For this review, take the finished solid that the model builds, in its own axes (mm). A direction names the side the tool comes from. Give positions to 0.01 mm unless a question says otherwise; leave off trailing zeros. Order: outer loops, then holes, each group sorted by start corner. A loop starts at its lowest first (then second) coordinate and runs counter-clockwise, first axis right, second up. Notation, with made-up numbers: (32.25, 68.25) - (58.25, 68.25) arc R21 ccw to (58.25, 83.25) - close; hole circle Ø4 at (79.5, 26.25). An arc over 180 degrees is marked (long way). Put each result on its own line as item: value. Start each with the question number.
```python
from build123d import *

# Parameters (mm, degrees)
BOSS_EXTRUDE1_DEPTH = 5
SKETCH2_R           = 2
CUT_EXTRUDE1_DEPTH  = 7
SKETCH3_R           = 2
CUT_EXTRUDE2_DEPTH  = 7
FILLET1_R           = 3


with BuildPart() as part:
    # Sketch1 → Boss-Extrude1 (new, symmetric)
    with BuildSketch(Plane.XY):
        with BuildLine():
            Line((0, 32), (0, 0))
            Line((0, 0), (8, 0))
            ThreePointArc((8, 0), (22.296085696, 3.651940128), (37, 4.880613018))
            ThreePointArc((37, 4.880613018), (49.464275388, 0.752368163), (57, -10))
            Line((57, -10), (65, -10))
            Line((65, -10), (65, 22))
            Line((65, 22), (57, 22))
            ThreePointArc((57, 22), (42.703914304, 18.348059872), (28, 17.119386982))
            ThreePointArc((28, 17.119386982), (15.535724612, 21.247631837), (8, 32))
            Line((8, 32), (0, 32))
        make_face()
    extrude(amount=BOSS_EXTRUDE1_DEPTH, both=True)

    # Sketch2 → Cut-Extrude1 (cut)
    with BuildSketch(Plane(origin=(65, 0, 0), x_dir=(0, 0, -1), z_dir=(1, 0, 0))):
        with Locations(Location((0, -2, 0), (0, 0, 90))):
            Circle(SKETCH2_R)
        with Locations(Location((0, 14, 0), (0, 0, 90))):
            Circle(SKETCH2_R)
    extrude(amount=-CUT_EXTRUDE1_DEPTH, mode=Mode.SUBTRACT)

    # Sketch3 → Cut-Extrude2 (cut)
    with BuildSketch(Plane.ZY):
        with Locations((0, 8)):
            Circle(SKETCH3_R)
        with Locations((0, 24)):
            Circle(SKETCH3_R)
    extrude(amount=-CUT_EXTRUDE2_DEPTH, mode=Mode.SUBTRACT)

    # Fillet1
    fillet1_edges = [part.edges().sort_by_distance(p)[0] for p in [
        (15.535724612, 21.247631837, -5),
        (42.703914304, 18.348059872, -5),
        (61, 22, -5),
        (61, -10, -5),
        (49.464275388, 0.752368163, -5),
        (22.296085696, 3.651940128, -5),
        (4, 0, 5),
        (4, 0, -5),
        (4, 32, -5),
        (22.296085696, 3.651940128, 5),
        (8, 32, 0),
        (57, 22, 0),
        (57, -10, 0),
        (8, 0, 0),
        (49.464275388, 0.752368163, 5),
        (61, -10, 5),
        (61, 22, 5),
        (42.703914304, 18.348059872, 5),
        (15.535724612, 21.247631837, 5),
        (4, 32, 5),
    ]]
    fillet(fillet1_edges, radius=FILLET1_R)


solid = part.part
```
1. Add section B-B, the plane y = 9. Give the boundary of the cut face in (x, z), then the cut area to 3 significant figures.
2. Wall thickness on line 1 (Y direction, x = 1.75, z = 0); line 2 (Z direction, x = 61.75, y = 14); line 3 (Y direction, x = 59, z = -0.5): over which ranges is each line inside the solid? List them lowest first. Write a range as from..to.
3. Add section D-D, the plane z = 4.25. Give the boundary of the cut face in (x, y), then the cut area to 3 significant figures.
4. Add section C-C, the plane z = -3.25. Give the boundary of the cut face in (x, y), then the cut area to 3 significant figures.
5. The part is to be moulded in two halves that separate along X. For faces 6 (the face through (42.66, 18.34, 0.03)), 7 (the face through (7, 8, 0)), 8 (the face through (58, -2, 0)), 9 (the face through (61.2, 21.1, 4.14)), say which applies: released by +X, released by -X, zero draft, split by the parting line, or undercut.
6. Clearance check with flat-ended pins moving along their axes: pin 1 (2 mm diameter, centred on y = 24, z = 0.5, fed in from -X); pin 2 (4.5 mm diameter, centred on x = 4, z = -1, fed in from -Y); pin 3 (4 mm diameter, centred on x = 45.5, z = 1.5, fed in from +Y). State where each tip first meets the part, or that it passes through.
7. Tool access review of faces 1 (the face through (7, 24, 0)), 2 (the face through (58, 14, 0)), 3 (the face through (4, 0, 0)), 4 (the face through (61.2, 21.1, -4.14)), 5 (the face through (22.34, 3.66, 0.03)): name each direction out of +Z, -Z, +X, -X, +Y, -Y from which nothing blocks a thin tool from reaching the whole face with its end or side.
Found:
1. outline: (0, -5) - (65, -5) - (65, 5) - (0, 5) - (0, 1.73) - (7, 1.73) - (7, -1.73) - (0, -1.73) - close
1. area: 626 mm^2
2. line 1: y = 0..6, 10..22, 26..32
2. line 2: z = -5..-2, 2..5
2. line 3: y = -10..-3.94, -0.06..12.06, 15.94..22
3. outline: (0, 1.02) - (7.5, 1.02) arc R1.98 ccw to (8.14, 1.12) arc R89.61 cw to (37, 5.9) arc R21.9 cw to (57.28, -7.75) arc R1.98 ccw to (59.12, -8.98) - (65, -8.98) - (65, 20.98) - (57.5, 20.98) arc R1.98 ccw to (56.86, 20.88) arc R89.61 cw to (28, 16.1) arc R21.9 cw to (7.72, 29.75) arc R1.98 ccw to (5.88, 30.98) - (0, 30.98) - close
3. area: 1,220 mm^2
4. outline: (0, 0.27) - (7.5, 0.27) arc R2.73 ccw to (8.38, 0.42) arc R88.87 cw to (37, 5.15) arc R21.15 cw to (56.59, -8.03) arc R2.73 ccw to (59.12, -9.73) - (65, -9.73) - (65, 21.73) - (57.5, 21.73) arc R2.73 ccw to (56.62, 21.58) arc R88.87 cw to (28, 16.85) arc R21.15 cw to (8.41, 30.03) arc R2.73 ccw to (5.88, 31.73) - (0, 31.73) - close
4. area: 1,320 mm^2
5. face 6: undercut
5. face 7: released by -X
5. face 8: released by +X
5. face 9: zero draft
6. pin 1: stops at x = 7
6. pin 2: stops at y = 0
6. pin 3: stops at y = 19.29
7. face 1: -X
7. face 2: +X
7. face 3: +Z, -Z, -X, -Y
7. face 4: -Z, +X, +Y
7. face 5: +Z, -Z, -Y
